from build123d import *

# Parameters (mm, degrees)
SKETCH_1_W          = 21
SKETCH_1_H          = 4
SKETCH_1_W_2        = 3
SKETCH_1_H_2        = 5
EXTRUDE_1_DEPTH     = 20
FILLET_1_R          = 10
FILLET_2_R          = 3
CUT_EXTRUDE_1_REACH = 51.399
SKETCH_2_R          = 2.25


with BuildPart() as part:
    # 草图1 → 凸台-拉伸1 (new body)
    with BuildSketch(Plane(origin=(0, 0, 0), x_dir=(1, 0, 0), z_dir=(0, 1, 0))):
        with BuildLine():
            Line((0, -4), (0, 0))
            Line((0, 0), (-3, 0))
            ThreePointArc((-3, 0), (-13.522200743, -8.125434387), (-19.5, -20))
            Line((-19.5, -20), (0, -20))
            Line((0, -20), (0, -4))
        make_face()
        with Locations((10.5, -2)):
            Rectangle(SKETCH_1_W, SKETCH_1_H)
        with Locations((-1.5, 2.5)):
            Rectangle(SKETCH_1_W_2, SKETCH_1_H_2)
        with Locations((22.5, 2.5)):
            Rectangle(SKETCH_1_W_2, SKETCH_1_H_2)
        with BuildLine():
            Line((24, 0), (21, 0))
            Line((21, 0), (21, -4))
            Line((21, -4), (21, -20))
            Line((21, -20), (40.5, -20))
            ThreePointArc((40.5, -20), (34.522200743, -8.125434387), (24, 0))
        make_face()
    extrude(amount=EXTRUDE_1_DEPTH)

    # 圆角1
    fillet_1_edges = [part.edges().sort_by_distance(p)[0] for p in [
        (21, 10, 4),
        (0, 10, 4),
    ]]
    fillet(fillet_1_edges, radius=FILLET_1_R)

    # 圆角2
    fillet_2_edges = [part.edges().sort_by_distance(p)[0] for p in [
        (24, 10, 0),
        (-3, 10, 0),
    ]]
    fillet(fillet_2_edges, radius=FILLET_2_R)

    # 草图2 → 切除-拉伸1 (cut, up to next)
    with BuildSketch(Plane(origin=(0, 0, 0), x_dir=(-1, 0, 0), z_dir=(0, 0, -1)), mode=Mode.PRIVATE) as cut_extrude_1_sk1:
        with Locations((-10.5, 10)):
            Circle(SKETCH_2_R)
    cut_extrude_1_tool1 = extrude(cut_extrude_1_sk1.sketch, amount=-CUT_EXTRUDE_1_REACH, mode=Mode.PRIVATE) & part.part
    add(cut_extrude_1_tool1.solids().sort_by_distance((10.5, 10, 0))[0], mode=Mode.SUBTRACT)


solid = part.part
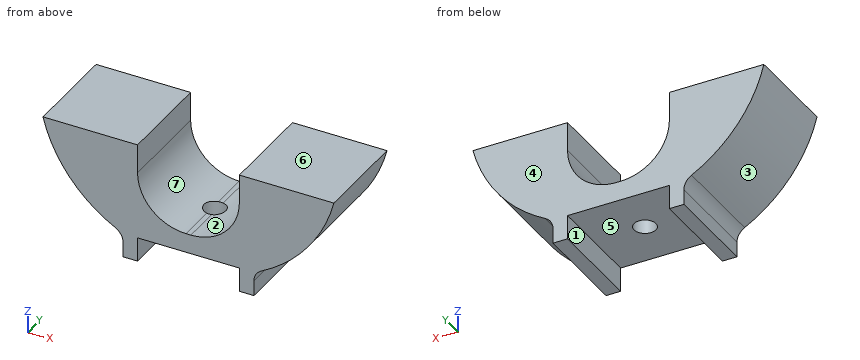
Input: part model. Units: mm. Frame: model coordinates. Face numbers are marked on the shaded views. A direction names the side the tool comes from. Coordinates: 2 decimals unless noted, no trailing zeros. Write each loop counter-clockwise with the first axis right and the second up, starting at its lowest first coordinate (ties: lowest second). Pieces come first, ordered by that corner, then holes. Notation, with made-up numbers: M 62,20.25 L 66,20.25 A11 cw 66,39.25 Z; hole C 10.25,33.5 d5. An arc over 180 degrees is marked long. Answer as a JSON object with one key per item and string values. Group by question number.
(1) Contact query for flat-ended pins moving along their axis: P1, Ø1.1, axis at x = 10.5, y = 3.5, coming from the +Z side; P2, Ø5.5, axis at y = 12.5, z = -2.5, coming from the -X side; P3, Ø2, axis at y = 4.5, z = 8.5, coming from the -X side. Output: stop coordinate, or through.
(2) Section A-A on y = 10. Output: boundary loops of the cut face in (x, z).
(3) Section B-B on z = -2.5. Output: boundary loops of the cut face in (x, y).
(4) Ray query, line 1 along Y through (x, z) = (10.5, 2.2); line 2 along X through (y, z) = (10, 2.25); line 3 along X through (y, z) = (10, 0.95). Return the intervals inside material, ascending. Write a range as [from, to].
(5) Section D-D on z = 5.5. Output: boundary loops of the cut face in (x, y), plus the area to 3 significant figures.
(6) Mould query, pull axis X, two halves, no side actions, for the marked faces 1, 2, 3 and 4. Classes: pulls with the +X half, pulls with the -X half, needs draft (parallel to the pull), parting line crosses it, or undercut.
(7) Section C-C on y = 17.75. Output: boundary loops of the cut face in (x, z).
(8) Set-up query: the marked faces 5, 6 and 7. Return all of +Z, -Z, +X, -X, +Y, -Y with unobstructed straight access to the full face (end or side cutting, diameter ignored); none if empty.
Result set:
{
 "1": {"P1": "stops at z = 4", "P2": "stops at x = -3.86", "P3": "stops at x = -14.59"},
 "2": {"outline": "M -19.5,20 A30 ccw -4.58,0.79 A3 cw -3,-1.85 L -3,-5 L 0,-5 L 0,0 L 8.25,0 L 8.25,4.15 A10 cw 0,14 L 0,20 Z; M 12.75,0 L 21,0 L 21,-5 L 24,-5 L 24,-1.85 A3 cw 25.58,0.79 A30 ccw 40.5,20 L 21,20 L 21,14 A10 cw 12.75,4.15 Z"},
 "3": {"outline": "M -3,0 L 0,0 L 0,20 L -3,20 Z; M 21,0 L 24,0 L 24,20 L 21,20 Z"},
 "4": {"line 1": "y = [0, 7.75], [12.25, 20]", "line 2": "x = [-7.01, 8.25], [12.75, 28.01]", "line 3": "x = [-4.87, 8.25], [12.75, 25.87]"},
 "5": {"outline": "M -11.08,0 L 4.73,0 L 4.73,20 L -11.08,20 Z; M 16.27,0 L 32.08,0 L 32.08,20 L 16.27,20 Z", "area": "632 mm2"},
 "6": {"face 1": "undercut", "face 2": "undercut", "face 3": "pulls with the -X half", "face 4": "needs draft"},
 "7": {"outline": "M -19.5,20 A30 ccw -4.58,0.79 A3 cw -3,-1.85 L -3,-5 L 0,-5 L 0,0 L 21,0 L 21,-5 L 24,-5 L 24,-1.85 A3 cw 25.58,0.79 A30 ccw 40.5,20 L 21,20 L 21,14 A10 cw 11,4 L 10,4 A10 cw 0,14 L 0,20 Z"},
 "8": {"face 5": "-Z, +Y, -Y", "face 6": "+Z, +X, -X, +Y, -Y", "face 7": "+Z, +Y, -Y"}
}
